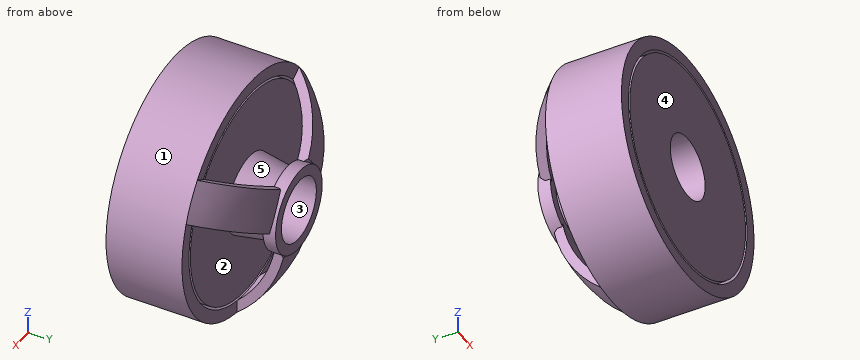
from build123d import *

# Parameters (mm, degrees)
SKETCH1_R           = 47.5
BOSS_EXTRUDE1_DEPTH = 30
SKETCH2_R           = 12.5
CUT_EXTRUDE1_DEPTH  = 30
SKETCH3_R           = 42.5
SKETCH3_R_2         = 41.5
CUT_EXTRUDE3_DEPTH  = 74.569694848
SKETCH6_R           = 13
SKETCH5_R           = 15.5
SKETCH9_R           = 12
CUT_EXTRUDE4_DEPTH  = 81.854808144
CIRPATTERN1_COUNT   = 3
SKETCH18_R          = 16.711627315
BOSS_EXTRUDE3_DEPTH = 5
SKETCH19_R          = 12.5
CUT_EXTRUDE5_DEPTH  = 84.740671179


with BuildPart() as part:
    # Sketch1 → Boss-Extrude1 (new body)
    with BuildSketch(Plane(origin=(0, 0, 0), x_dir=(1, 0, 0), z_dir=(0, 1, 0))):
        with Locations(Location((0, 0, 0), (0, 0, 270))):
            Circle(SKETCH1_R)
    extrude(amount=BOSS_EXTRUDE1_DEPTH)

    # Sketch2 → Cut-Extrude1 (cut)
    with BuildSketch(Plane(origin=(0, 30, 0), x_dir=(1, 0, 0), z_dir=(0, 1, 0))):
        with Locations(Location((0, 0, 0), (0, 0, 270))):
            Circle(SKETCH2_R)
    extrude(amount=-CUT_EXTRUDE1_DEPTH, mode=Mode.SUBTRACT)

    # Sketch3 → Cut-Extrude3 (cut, through all)
    with BuildSketch(Plane(origin=(0, 30, 0), x_dir=(1, 0, 0), z_dir=(0, 1, 0))):
        with Locations(Location((0, 0, 0), (0, 0, 270))):
            Circle(SKETCH3_R)
        with Locations(Location((0, 0, 0), (0, 0, 270))):
            Circle(SKETCH3_R_2, mode=Mode.SUBTRACT)
    extrude(amount=-CUT_EXTRUDE3_DEPTH, mode=Mode.SUBTRACT)


with BuildPart() as cut_extrude3_piece_1:
    # of the separate pieces the step leaves, piece 1, a body of its own (cut_extrude3_pieces)
    add(part.part.solids().sort_by_distance((0, 0, 41.5))[0])

    # Sketch6 → Loft1 section 0
    with BuildSketch(Plane(origin=(0, 45, 0), x_dir=(-1, 0, 0), z_dir=(0, -1, 0))):
        Circle(SKETCH6_R)
    # Sketch5 → Loft1 section 1
    with BuildSketch(Plane(origin=(0, 30, 0), x_dir=(1, 0, 0), z_dir=(0, 1, 0))):
        Circle(SKETCH5_R)
    loft()

    # Sketch9 → Cut-Extrude4 (cut, through all)
    with BuildSketch(Plane(origin=(0, 45, 0), x_dir=(1, 0, 0), z_dir=(0, 1, 0))):
        with Locations(Location((0, 0, 0), (0, 0, 270))):
            Circle(SKETCH9_R)
    extrude(amount=-CUT_EXTRUDE4_DEPTH, mode=Mode.SUBTRACT)



with BuildPart() as cut_extrude3_piece_2:
    # of the separate pieces the step leaves, piece 2, a body of its own (cut_extrude3_pieces)
    add(part.part.solids().sort_by_distance((0, 0, 47.5))[0])

    # Sweep1: sweep along a path in Sketch13
    with BuildLine(Plane(origin=(0, 0, 0), x_dir=(0, 0, -1), z_dir=(1, 0, 0))) as sweep1_path:
        ThreePointArc((12, 45), (28.013623807, 39.985126821), (41.5, 30))
    # Sketch10 → Sweep1 (sweep)
    with BuildSketch(Plane(origin=(0, 30, 0), x_dir=(1, 0, 0), z_dir=(0, 1, 0))):
        with BuildLine():
            Line((8.039798927, 41.732620733), (8.039798927, 46.814651907))
            ThreePointArc((8.039798927, 46.814651907), (0, 47.5), (-8.039798927, 46.814651907))
            Line((-8.039798927, 46.814651907), (-8.039798927, 41.732620733))
            ThreePointArc((-8.039798927, 41.732620733), (0, 42.5), (8.039798927, 41.732620733))
        make_face()
    sweep1 = sweep(path=sweep1_path.line)

    # CirPattern1: Sweep1 ×3 about axis
    cirpattern1_axis = Axis((0, 30, 0), (0, 1, 0))
    for i in range(1, CIRPATTERN1_COUNT):
        add(sweep1.rotate(cirpattern1_axis, i * 360 / CIRPATTERN1_COUNT))


with BuildPart() as cut_extrude3_piece_1_1:
    add(cut_extrude3_piece_1.part)

    add(cut_extrude3_piece_2.part)  # Boss-Extrude3 merges Cut-Extrude3 piece 2
    # Sketch18 → Boss-Extrude3 (add)
    with BuildSketch(Plane(origin=(0, 50, 0), x_dir=(-1, 0, 0), z_dir=(0, -1, 0))):
        with Locations(Location((0, 0, 0), (0, 0, 90))):
            Circle(SKETCH18_R)
    extrude(amount=BOSS_EXTRUDE3_DEPTH)

    # Sketch19 → Cut-Extrude5 (cut, through all)
    with BuildSketch(Plane(origin=(0, 50, 0), x_dir=(1, 0, 0), z_dir=(0, 1, 0))):
        with Locations(Location((0, 0, 0), (0, 0, 270))):
            Circle(SKETCH19_R)
    extrude(amount=-CUT_EXTRUDE5_DEPTH, mode=Mode.SUBTRACT)


solid = cut_extrude3_piece_1_1.part
Design review of the part built by this model. Coordinates are the model's own, in mm. Face numbers are marked on the shaded views. A direction names the side the tool comes from. Round coordinates to 2 decimals unless told otherwise and drop trailing zeros. Loops run counter-clockwise (first coordinate to the right, second up) from the corner with the lowest first, then second, coordinate; pieces in that order, holes last. Notation, with made-up numbers: (-25, 52) - (-8, 52) arc R18 ccw to (-8, 86) - close; hole circle Ø6 at (51.5, 61.25). An arc over 180 degrees is marked (long way). One line per item, written item: value. Start each with the question number.
1) For the marked faces 1 and 2, list the 3-axis set-ups (+Z, -Z, +X, -X, +Y, -Y) from which the entire face can be reached by the end or side of a thin tool; tool diameter is ignored.
2) To check wall thickness, follow L1, parallel to X at y = 22, z = 0; L2, parallel to Z at x = 17, y = 10.5; L3, parallel to X at y = 17, z = 14. State the ranges of each line that lie inside material, in increasing order. Write a range as from..to.
3) Consider section C-C on x = 28. Give the number of separate pieces and of enclosed holes in the cut face, then the cut area to 3 significant figures.
4) Consider section B-B on z = 35. Give the boundary of the cut face in (x, y), then the cut area to 3 significant figures.
5) Insertion check: pin 1 Ø12 at (x, z) = (25.5, -11) entering from +Y; pin 2 Ø5 at (y, z) = (6, 3.5) entering from -X; pin 3 Ø8 at (y, z) = (18, -35.5) entering from +X. Each pin has a flat end and moves straight along its axis. Give the tip position at first contact, or say it passes through.
6) Consider section A-A on y = 20. Give the boundary of the cut face in (x, z).
7) Draft analysis for pull direction Y (two halves, no side actions). For the marked faces 3, 4 and 5, state which applies: +Y half, -Y half, draft (parallel to the pull), parting line (faces both ways), or undercut.
Reported:
1. face 1: +Y, -Y
1. face 2: none
2. L1: x = -47.5..-42.5, -41.5..-12.5, 12.5..41.5, 42.5..47.5
2. L2: z = -44.35..-38.95, -37.86..37.86, 38.95..44.35
2. L3: x = -45.39..-40.13, -39.07..39.07, 40.13..45.39
3. separate pieces: 4
3. enclosed holes: 0
3. area: 2,300 mm^2
4. outline: (-32.11, 0) - (-24.11, 0) - (-24.11, 30) - (-32.11, 30) - close; (-22.3, 0) - (22.3, 0) - (22.3, 30) - (-22.3, 30) - close; (24.11, 0) - (32.11, 0) - (32.11, 30) - (24.11, 30) - close
4. area: 1,820 mm^2
5. pin 1: stops at y = 30
5. pin 2: stops at x = -47.49
5. pin 3: stops at x = 35.55
6. outline: circle Ø95 at (0, 0); circle Ø83 at (0, 0); hole circle Ø85 at (0, 0); hole circle Ø25 at (0, 0)
7. face 3: draft
7. face 4: -Y half
7. face 5: undercut
